Read the model definition and answer for the solid it produces. Units are mm, in the model's axes. A direction names the side the tool comes from. Coordinates: 2 decimals unless noted, no trailing zeros. Write each loop counter-clockwise with the first axis right and the second up, starting at its lowest first coordinate (ties: lowest second). Pieces come first, ordered by that corner, then holes.
(1) Section D-D on x = -63 is taken. Write down the section's boundary in (y, z), then the cut area to 3 significant figures.
(2) Section A-A on z = 0 is taken. Write down the section's boundary in (x, y), then the cut area to 3 significant figures.
(3) Given pin 1 (2 mm diameter, centred on x = 17.5, z = 1, fed in from +Y); pin 2 (15.5 mm diameter, centred on x = -6, y = 20, fed in from +Z); pin 3 (12 mm diameter, centred on y = 116.5, z = -28, fed in from -X), each flat-ended and moving along its own axis, determine where each tip first touches the part or whether it passes through.
(4) Find the intervals of material crossed by probe 1 along Z at (x, y) = (-101.6, 4.75); probe 2 along Y at (x, z) = (122, 0); probe 3 along Y at (x, z) = (125, -43.18), in increasing order.
(5) Which of the six approach directions +Z, -Z, +X, -X, +Y, -Y give full straight-line access (tool end or side, diameter ignored) to faces 5 (the flat face through (86, 43, -69.85)), 6 (the flat face through (75, 47, -76.2)), 7 (the flat face through (6.35, 14, 0))?
(6) Section C-C on y = 113.03 is taken. Write down the section's boundary in (x, z).
(7) The mould has two halves that part along Z. Classify faces 1 (the flat face through (86, 43, 69.85)), 2 (the flat face through (-19.05, 14, 0)), 3 (the flat face through (75, 47, 76.2)), 4 (the cylindrical face through (123.87, 22.84, 41.19)): +Z half, -Z half, draft (parallel to the pull), parting line (faces both ways), or undercut.
(8) Section B-B on y = 83 is taken. Write down the section's boundary in (x, z).
from build123d import *

# Parameters (mm, degrees)
SKETCH1_W           = 254
SKETCH1_H           = 152.4
BOSS_EXTRUDE1_DEPTH = 6.35
SKETCH2_W           = 152.4
SKETCH2_H           = 127
SKETCH2_R           = 50.8
SKETCH2_R_2         = 4.318
BOSS_EXTRUDE2_DEPTH = 6.35
BOSS_EXTRUDE3_DEPTH = 6.35
BOSS_EXTRUDE4_DEPTH = 6.35
SKETCH5_W           = 25.4
SKETCH5_H           = 50.8
BOSS_EXTRUDE5_DEPTH = 25.4
SKETCH6_R           = 50.8
CUT_EXTRUDE1_DEPTH  = 25.4
SKETCH7_R           = 6.35
CUT_EXTRUDE2_DEPTH  = 25.4


with BuildPart() as part:
    # Sketch1 → Boss-Extrude1 (new body)
    with BuildSketch(Plane(origin=(0, 0, 0), x_dir=(1, 0, 0), z_dir=(0, 1, 0))):
        Rectangle(SKETCH1_W, SKETCH1_H)
    extrude(amount=BOSS_EXTRUDE1_DEPTH)

    # Sketch2 → Boss-Extrude2 (add)
    with BuildSketch(Plane(origin=(127, 0, 0), x_dir=(0, 0, -1), z_dir=(1, 0, 0))):
        with Locations((0, 69.85)):
            Rectangle(SKETCH2_W, SKETCH2_H)
        with Locations((0, 69.85)):
            Circle(SKETCH2_R, mode=Mode.SUBTRACT)
        with Locations((-43.18, 26.67)):
            Circle(SKETCH2_R_2, mode=Mode.SUBTRACT)
        with Locations((43.18, 26.67)):
            Circle(SKETCH2_R_2, mode=Mode.SUBTRACT)
        with Locations((43.18, 113.03)):
            Circle(SKETCH2_R_2, mode=Mode.SUBTRACT)
        with Locations((-43.18, 113.03)):
            Circle(SKETCH2_R_2, mode=Mode.SUBTRACT)
    extrude(amount=-BOSS_EXTRUDE2_DEPTH)

    # Sketch3 → Boss-Extrude3 (add)
    with BuildSketch(Plane.XY.offset(76.2)):
        Polygon((120.65, 133.35), (0, 6.35), (120.65, 6.35), align=None)
    extrude(amount=-BOSS_EXTRUDE3_DEPTH)

    # Sketch4 → Boss-Extrude4 (add)
    with BuildSketch(Plane(origin=(0, 0, -76.2), x_dir=(-1, 0, 0), z_dir=(0, 0, -1))):
        Polygon((-120.65, 133.35), (0, 6.35), (-120.65, 6.35), align=None)
    extrude(amount=-BOSS_EXTRUDE4_DEPTH)

    # Sketch5 → Boss-Extrude5 (add)
    with BuildSketch(Plane(origin=(0, 6.35, 0), x_dir=(1, 0, 0), z_dir=(0, 1, 0))):
        with Locations((-6.35, 0)):
            Rectangle(SKETCH5_W, SKETCH5_H)
    extrude(amount=BOSS_EXTRUDE5_DEPTH)

    # Sketch6 → Cut-Extrude1 (cut)
    with BuildSketch(Plane.ZY.offset(19.05)):
        with Locations((0, 69.85)):
            Circle(SKETCH6_R)
    extrude(amount=-CUT_EXTRUDE1_DEPTH, mode=Mode.SUBTRACT)

    # Sketch7 → Cut-Extrude2 (cut)
    with BuildSketch(Plane(origin=(0, 6.35, 0), x_dir=(1, 0, 0), z_dir=(0, 1, 0))):
        with Locations((-101.6, 50.8)):
            Circle(SKETCH7_R)
        with Locations((-101.6, -50.8)):
            Circle(SKETCH7_R)
        with Locations((76.2, -50.8)):
            Circle(SKETCH7_R)
        with Locations((76.2, 50.8)):
            Circle(SKETCH7_R)
    extrude(amount=-CUT_EXTRUDE2_DEPTH, mode=Mode.SUBTRACT)


solid = part.part
Response:
1. outline: (0, -76.2) - (6.35, -76.2) - (6.35, 76.2) - (0, 76.2) - close
1. area: 968 mm2
2. outline: (-127, 0) - (127, 0) - (127, 19.05) - (120.65, 19.05) - (120.65, 6.35) - (6.35, 6.35) - (6.35, 19.05) - (-19.05, 19.05) - (-19.05, 6.35) - (-127, 6.35) - close; (120.65, 120.65) - (127, 120.65) - (127, 133.35) - (120.65, 133.35) - close
2. area: 2,100 mm2
3. pin 1: stops at y = 6.35
3. pin 2: stops at z = 25.4
3. pin 3: stops at x = 120.65
4. probe 1: z = -76.2 to -57.15, -44.45 to 44.45, 57.15 to 76.2
4. probe 2: y = 0 to 19.05, 120.65 to 133.35
4. probe 3: y = 0 to 22.35, 30.99 to 43.09, 96.61 to 108.71, 117.35 to 133.35
5. face 5: -X, +Y
5. face 6: -Z, +X, -X, +Y, -Y
5. face 7: +Y
6. outline: (101.35, -76.2) - (127, -76.2) - (127, -47.5) - (120.65, -47.5) - (120.65, -69.85) - (101.35, -69.85) - close; (101.35, 69.85) - (120.65, 69.85) - (120.65, 47.5) - (127, 47.5) - (127, 76.2) - (101.35, 76.2) - close; (120.65, -38.86) - (127, -38.86) - (127, -26.76) - (120.65, -26.76) - close; (120.65, 26.76) - (127, 26.76) - (127, 38.86) - (120.65, 38.86) - close
7. face 1: undercut
7. face 2: draft
7. face 3: +Z half
7. face 4: undercut
8. outline: (72.82, -76.2) - (127, -76.2) - (127, -49.07) - (120.65, -49.07) - (120.65, -69.85) - (72.82, -69.85) - close; (72.82, 69.85) - (120.65, 69.85) - (120.65, 49.07) - (127, 49.07) - (127, 76.2) - (72.82, 76.2) - close
